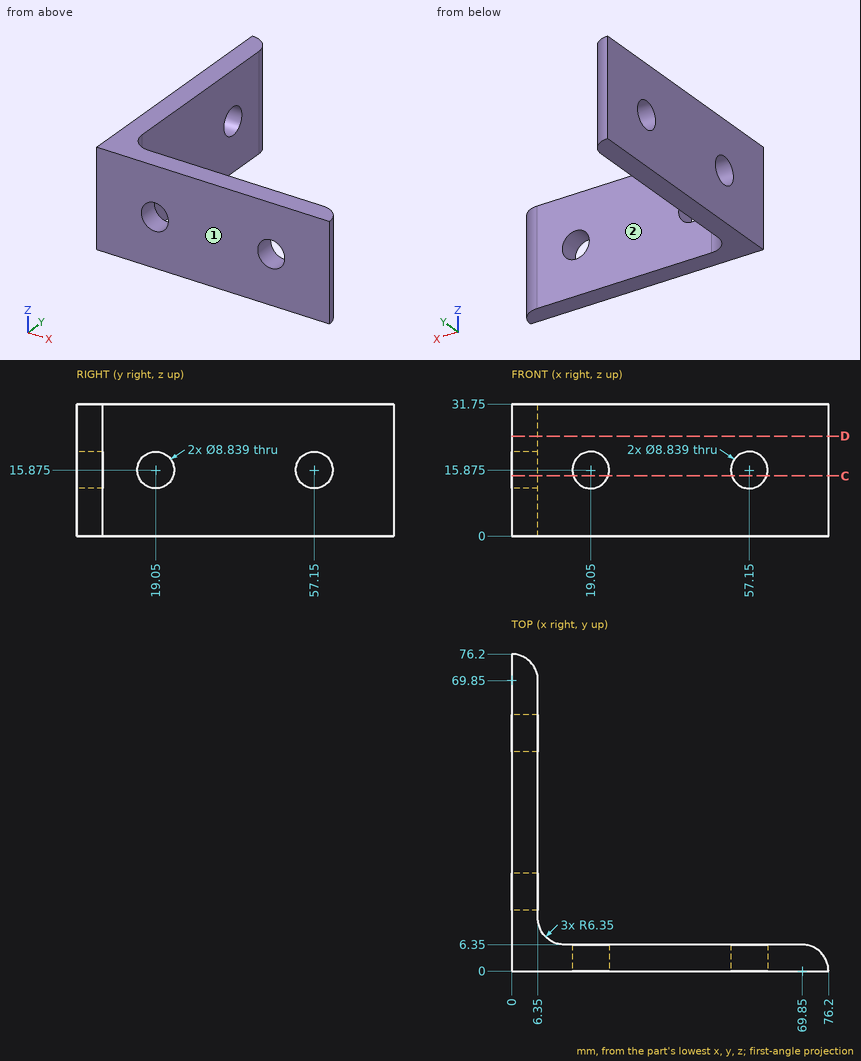
Geometry: see drawing. Coordinates: mm, zero at the bounding-box minimum. A direction names the side the tool comes from. Coordinates: 2 decimals unless noted, no trailing zeros. Loops run counter-clockwise (first coordinate to the right, second up) from the corner with the lowest first, then second, coordinate; pieces in that order, holes last.
(1) First-contact query: pin 1 Ø5.5 at (y, z) = (19.05, 15.875) entering from +X; pin 2 Ø16 at (x, z) = (33, 13.5) entering from +Y; pin 3 Ø16 at (y, z) = (43.5, 11.5) entering from +X. Flat tips, straight axial feed; report the tip coordinate or a pass-through.
(2) Section D-D on z = 24. Return the cut outline in (x, y), then the cut area to 3 significant figures.
(3) Section C-C on z = 14.5. Return the cut outline in (x, y).
(4) Set-up query: the marked faces 1 and 2. Return all of +Z, -Z, +X, -X, +Y, -Y with unobstructed straight access to the full face (end or side cutting, diameter ignored); none if empty.
(5) Material intervals for probe 1 along Z at (x, y) = (4, 57); probe 2 along X at (y, z) = (40, 18.5), sorted ascending.
Data:
1. pin 1: passes through
1. pin 2: stops at y = 6.35
1. pin 3: stops at x = 6.35
2. outline: (0, 0) - (76.2, 0) arc R6.35 ccw to (69.85, 6.35) - (12.7, 6.35) arc R6.35 cw to (6.35, 12.7) - (6.35, 69.85) arc R6.35 ccw to (0, 76.2) - close
2. area: 919 mm2
3. outline: (0, 0) - (14.85, 0) - (14.85, 6.35) - (12.7, 6.35) arc R6.35 cw to (6.35, 12.7) - (6.35, 14.85) - (0, 14.85) - close; (0, 23.25) - (6.35, 23.25) - (6.35, 52.95) - (0, 52.95) - close; (0, 61.35) - (6.35, 61.35) - (6.35, 69.85) arc R6.35 ccw to (0, 76.2) - close; (23.25, 0) - (52.95, 0) - (52.95, 6.35) - (23.25, 6.35) - close; (61.35, 0) - (76.2, 0) arc R6.35 ccw to (69.85, 6.35) - (61.35, 6.35) - close
4. face 1: +Z, -Z, +X, -X, -Y
4. face 2: +Z, -Z, +X, +Y
5. probe 1: z = 0 to 11.46, 20.29 to 31.75
5. probe 2: x = 0 to 6.35
